The model under review builds one solid part; all positions refer to its coordinate system, in mm. Face numbers are marked on the shaded views. A direction names the side the tool comes from. Give positions to 0.01 mm unless a question says otherwise; leave off trailing zeros. Order: outer loops, then holes, each group sorted by start corner. A loop starts at its lowest first (then second) coordinate and runs counter-clockwise, first axis right, second up. Notation, with made-up numbers: (77.25, 65) - (82.25, 65) arc R16 cw to (82.25, 86) - close; hole circle Ø1 at (10, 83). An arc over 180 degrees is marked (long way). Put each result on its own line as item: value.
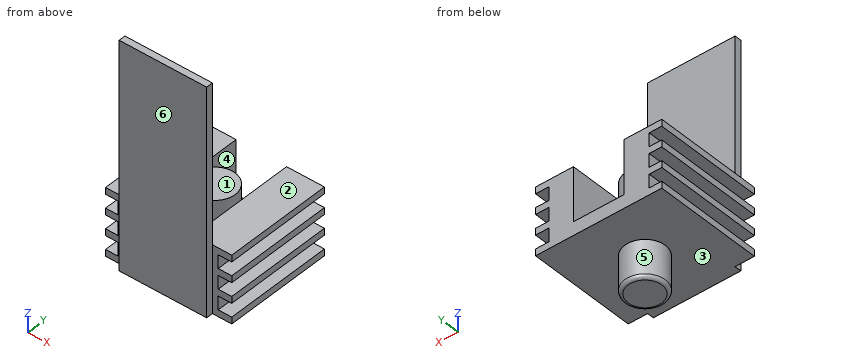
```python
from build123d import *

# Parameters (mm, degrees)
F0_W      = 37.5
F0_H      = 32.25
F1_DEPTH  = 20
F2_R      = 6
F3_DEPTH  = 11
F4_W      = 15
F4_H      = 16
F4_W_2    = 3.7276374176
F4_H_2    = 4
F4_W_3    = 4.0285747498
F5_DEPTH  = 32.251
F6_R      = 1
F7_R      = 6
F8_DEPTH  = 17
F9_W      = 26
F9_H      = 2
F10_DEPTH = 67


with BuildPart() as f1:
    # F0 (on Top) → F1 (new body)
    with BuildSketch(Plane.XY):
        Rectangle(F0_W, F0_H)
    extrude(amount=F1_DEPTH)

    # F2 (on face) → F3 (join)
    with BuildSketch(Plane(origin=(0, 0, 0), x_dir=(1, 0, 0), z_dir=(0, 0, -1))):
        Circle(F2_R)
    extrude(amount=F3_DEPTH)

    # F4 (on face) → F5 (cut, through all)
    with BuildSketch(Plane.XZ.offset(16.125)):
        with Locations((0, 12)):
            Rectangle(F4_W, F4_H)
        with Locations((-16.8861812912, 16)):
            Rectangle(F4_W_2, F4_H_2)
        with Locations((-16.8861812912, 4)):
            Rectangle(F4_W_2, F4_H_2)
        with Locations((16.7357126251, 16)):
            Rectangle(F4_W_3, F4_H_2)
        with Locations((16.7357126251, 10)):
            Rectangle(F4_W_3, F4_H_2)
        with Locations((16.7357126251, 4)):
            Rectangle(F4_W_3, F4_H_2)
        with Locations((-16.8861812912, 10)):
            Rectangle(F4_W_2, F4_H_2)
    extrude(amount=-F5_DEPTH, mode=Mode.SUBTRACT)

    # F6
    f6_edges = [f1.edges().sort_by_distance(p)[0] for p in [
        (-6, 0, -11),
    ]]
    fillet(f6_edges, radius=F6_R)

    # F7 (on face) → F8 (join)
    with BuildSketch(Plane.XY.offset(4)):
        Circle(F7_R)
    extrude(amount=F8_DEPTH)

    # F9 (on Top) → F10 (join)
    with BuildSketch(Plane.XY):
        with Locations((0, -17.125)):
            Rectangle(F9_W, F9_H)
    extrude(amount=F10_DEPTH)


solid = f1.part
```
(1) Wall thickness on L1, parallel to Z at x = 16, y = -11.5; L2, parallel to X at y = -11, z = 7; L3, parallel to Z at x = -2.5, y = -6.5: over which ranges is each line inside the solid? List them lowest first.
The answers:
L1: 0 to 2, 6 to 8, 12 to 14, 18 to 20
L2: -18.75 to -7.5, 7.5 to 18.75
L3: 0 to 4
(2) Take a section at D-D, the plane x = 0. Write out the cut boundary in (y, z) (3 decimals).
The answers:
outline: (-18.125, 0) - (-6, 0) - (-6, -10) arc R1 ccw to (-5, -11) - (5, -11) arc R1 ccw to (6, -10) - (6, 0) - (16.125, 0) - (16.125, 4) - (6, 4) - (6, 21) - (-6, 21) - (-6, 4) - (-16.125, 4) - (-16.125, 67) - (-18.125, 67) - close
(3) For the marked faces 1, 2 and 3, list the 3-axis set-ups (+Z, -Z, +X, -X, +Y, -Y) from which the entire face can be reached by the end or side of a thin tool; tool diameter is ignored.
The answers:
face 1: +Z, +X, -X, +Y
face 2: +Z, +X, +Y
face 3: -Z
(4) The part is to be moulded in two halves that separate along X. For the marked faces 4, 5 and 6, say which applies: pulls with the +X half, pulls with the -X half, needs draft (parallel to the pull), parting line crosses it, or undercut.
The answers:
face 4: undercut
face 5: parting line crosses it
face 6: needs draft
(5) Take a section at A-A, the plane x = 11. Write out the cut boundary in (y, z) (3 decimals).
The answers:
outline: (-18.125, 0) - (16.125, 0) - (16.125, 20) - (-16.125, 20) - (-16.125, 67) - (-18.125, 67) - close
(6) Clearance check with flat-ended pins moving along their axes: pin 1 Ø2 at (x, y) = (17.5, 2.5) entering from +Z; pin 2 Ø1.2 at (y, z) = (5, 16) entering from +X; pin 3 Ø1.2 at (y, z) = (4, 15.5) entering from -X. State where each tip first meets the part, or that it passes through.
The answers:
pin 1: z = 20
pin 2: x = 14.72
pin 3: x = -15.02
(7) Take a section at C-C, the plane z = 49. Write out the cut boundary in (x, y) (3 decimals).
The answers:
outline: (-13, -18.125) - (13, -18.125) - (13, -16.125) - (-13, -16.125) - close
